Can you work these out from the model? Positions are in its coordinate system, mm. A direction names the side the tool comes from. Round coordinates to 2 decimals unless told otherwise and drop trailing zeros. Write each loop counter-clockwise with the first axis right and the second up, starting at its lowest first coordinate (ties: lowest second). Pieces come first, ordered by that corner, then holes.
Q1. For faces 1 (the cylindrical face through (4.721, -13.559, 23.554)), 2 (the cylindrical face through (4.721, 27.178, -0.034)), 3 (the cylindrical face through (4.721, -15.875, 0.115)), which set-ups out of +Z, -Z, +X, -X, +Y, -Y let a thin tool reach every point of the face, with its end or its side?
Q2. I'm going to push flat-ended pins straight in: pin 1 Ø2 at (x, y) = (10.5, 21) entering from -Z; pin 2 Ø12 at (x, z) = (18.5, 2.5) entering from -Y; pin 3 Ø5.5 at (x, y) = (4, 22.5) entering from -Z; pin 4 Ø4 at (y, z) = (10.32, -17.87) entering from -X. Where does each tip first touch, or does it pass through?
Q3. If we section it at A-A (z = 0): Give the number of separate pieces and of enclosed holes in the cut face, plus the area to 3 significant figures.
Q4. If we section it at B-B (x = 17.75): Please give me the cut outline in (y, z).
Q5. If we section it at D-D (y = -21.5): Please give me the cut outline in (x, z), plus the area to 3 significant figures.
Q6. Please list where these lines run through material, in increasing order: line 1 along Y through (x, z) = (24.45, 0); line 2 along Y through (x, z) = (27, 0); line 3 along Y through (x, z) = (10.65, 0).
from build123d import *

# Parameters (mm, degrees)
MOUNTING_HOLE_D               = 4.9149
CIRPATTERN1_COUNT             = 3
SKETCH26_R                    = 15.1511
SKETCH26_R_2                  = 12.0396
AXIAL_O_RING_GLAND_DEPTH      = 1.9558
PRESSURE_TAP_CLEARANCE_HOLE_D = 12.7
THERMOCOUPLE_CLEARANCE_HOLE_D = 4.9149
SKETCH7_R                     = 34.7345
CUT_EXTRUDE1_DEPTH            = 9.5758
FILLET1_R                     = 2.54
FILLET2_R                     = 6.604


with BuildPart() as part:
    # Sketch1 → Revolve2 (revolve)
    with BuildSketch(Plane.XY, mode=Mode.PRIVATE) as revolve2_sk:
        Polygon((27.94, 34.671), (9.5758, 34.671), (9.5758, 27.94), (0, 27.94), (0, 0), (25.4, 0), (25.4, 29.2608), (27.94, 29.2608), align=None)
    revolve(revolve2_sk.sketch.rotate(Axis((-88.99, 0, 0), (1, 0, 0)), 90), axis=Axis((-88.99, 0, 0), (1, 0, 0)))

    # Sketch28 → NPT Center Bore (revolve, cut)
    with BuildSketch(Plane.ZX):
        Polygon((0, 0), (0, 27.94), (5.5626, 27.94), (5.5626, 10.16), (6.557974294, 10.16), (6.8621783, 0), align=None)
    revolve(axis=Axis((-6.35, 0, 0), (1, 0, 0)), mode=Mode.SUBTRACT)

    # Mounting Hole (through all)
    with Locations(Plane.ZY):
        with Locations((0, 20.6375)):
            mounting_hole = Hole(MOUNTING_HOLE_D / 2)

    # CirPattern1: Mounting Hole ×3 about axis
    cirpattern1_axis = Axis((0, 0, 0), (1, 0, 0))
    for i in range(1, CIRPATTERN1_COUNT):
        add(mounting_hole.rotate(cirpattern1_axis, i * 360 / CIRPATTERN1_COUNT), mode=Mode.SUBTRACT)

    # Sketch26 → Axial O-Ring Gland (cut)
    with BuildSketch(Plane(origin=(25.4, 0, 0), x_dir=(0, 0, -1), z_dir=(1, 0, 0))):
        Circle(SKETCH26_R)
        Circle(SKETCH26_R_2, mode=Mode.SUBTRACT)
    extrude(amount=-AXIAL_O_RING_GLAND_DEPTH, mode=Mode.SUBTRACT)

    # Sketch30 → Flow Cone (revolve, cut)
    with BuildSketch(Plane.XY, mode=Mode.PRIVATE) as flow_cone_sk:
        Polygon((11.093885077, 5.5626), (25.4, 10.7696), (25.4, 5.5626), align=None)
    revolve(flow_cone_sk.sketch.rotate(Axis((-88.99, 0, 0), (1, 0, 0)), 90), axis=Axis((-88.99, 0, 0), (1, 0, 0)), mode=Mode.SUBTRACT)

    # Pressure Tap Clearance Hole (through all)
    with Locations(Plane.ZY):
        with Locations((19.247414599, 11.1125)):
            Hole(PRESSURE_TAP_CLEARANCE_HOLE_D / 2)

    # Thermocouple Clearance Hole (through all)
    with Locations(Plane.ZY):
        with Locations((-17.872599271, 10.31875)):
            Hole(THERMOCOUPLE_CLEARANCE_HOLE_D / 2)

    # Sketch7 → Cut-Extrude1 (cut)
    with BuildSketch(Plane.ZY):
        Circle(SKETCH7_R)
        with BuildLine():
            Line((15.496152366, -3.447446426), (25.553900006, -9.254289733))
            ThreePointArc((25.553900006, -9.254289733), (23.536838424, -13.589), (20.791400006, -17.503181704))
            Line((20.791400006, -17.503181704), (10.733652366, -11.696338397))
            ThreePointArc((10.733652366, -11.696338397), (0, -15.875), (-10.733652366, -11.696338397))
            Line((-10.733652366, -11.696338397), (-20.791400006, -17.503181704))
            ThreePointArc((-20.791400006, -17.503181704), (-23.536838424, -13.589), (-25.553900006, -9.254289733))
            Line((-25.553900006, -9.254289733), (-15.496152366, -3.447446426))
            ThreePointArc((-15.496152366, -3.447446426), (-13.748153285, 7.9375), (-4.7625, 15.143784822))
            Line((-4.7625, 15.143784822), (-4.7625, 26.757471438))
            ThreePointArc((-4.7625, 26.757471438), (0, 27.178), (4.7625, 26.757471438))
            Line((4.7625, 26.757471438), (4.7625, 15.143784822))
            ThreePointArc((4.7625, 15.143784822), (13.748153285, 7.9375), (15.496152366, -3.447446426))
        make_face(mode=Mode.SUBTRACT)
    extrude(amount=-CUT_EXTRUDE1_DEPTH, mode=Mode.SUBTRACT)

    # Fillet1
    fillet1_edges = [part.edges().sort_by_distance(p)[0] for p in [
        (4.7879, -9.254289733, 25.553900006),
        (4.7879, -17.503181704, 20.791400006),
        (4.7879, -17.503181704, -20.791400006),
        (4.7879, -9.254289733, -25.553900006),
        (4.7879, 26.757471438, -4.7625),
        (4.7879, 26.757471438, 4.7625),
    ]]
    fillet(fillet1_edges, radius=FILLET1_R)

    # Fillet2
    fillet2_edges = [part.edges().sort_by_distance(p)[0] for p in [
        (4.7879, -3.447446426, 15.496152366),
        (4.7879, -11.696338397, 10.733652366),
        (4.7879, -11.696338397, -10.733652366),
        (4.7879, -3.447446426, -15.496152366),
        (4.7879, 15.143784822, -4.7625),
        (4.7879, 15.143784822, 4.7625),
    ]]
    fillet(fillet2_edges, radius=FILLET2_R)


solid = part.part
A:
1. face 1: +Z, -X, -Y
1. face 2: -X, +Y
1. face 3: -X, -Y
2. pin 1: stops at z = -28.32
2. pin 2: stops at y = -34.67
2. pin 3: stops at z = -4.76
2. pin 4: passes through
3. separate pieces: 3
3. enclosed holes: 0
3. area: 1,020 mm2
4. outline: circle Ø69.34 at (0, 0); hole circle Ø4.91 at (-10.32, -17.87); hole circle Ø4.91 at (-10.32, 17.87); hole circle Ø15.97 at (0, 0); hole circle Ø12.7 at (11.11, 19.25); hole circle Ø4.91 at (10.32, -17.87); hole circle Ø4.91 at (20.64, 0)
5. outline: (9.58, -27.2) - (27.94, -27.2) - (27.94, -19.85) - (25.4, -19.85) - (25.4, 19.85) - (27.94, 19.85) - (27.94, 27.2) - (9.58, 27.2) - close
5. area: 898 mm2
6. line 1: y = -34.67 to -15.15, -12.04 to -10.42, 10.42 to 12.04, 15.15 to 18.18, 23.09 to 34.67
6. line 2: y = -34.67 to -29.26, 29.26 to 34.67
6. line 3: y = -34.67 to -5.56, 5.56 to 18.18, 23.09 to 34.67
